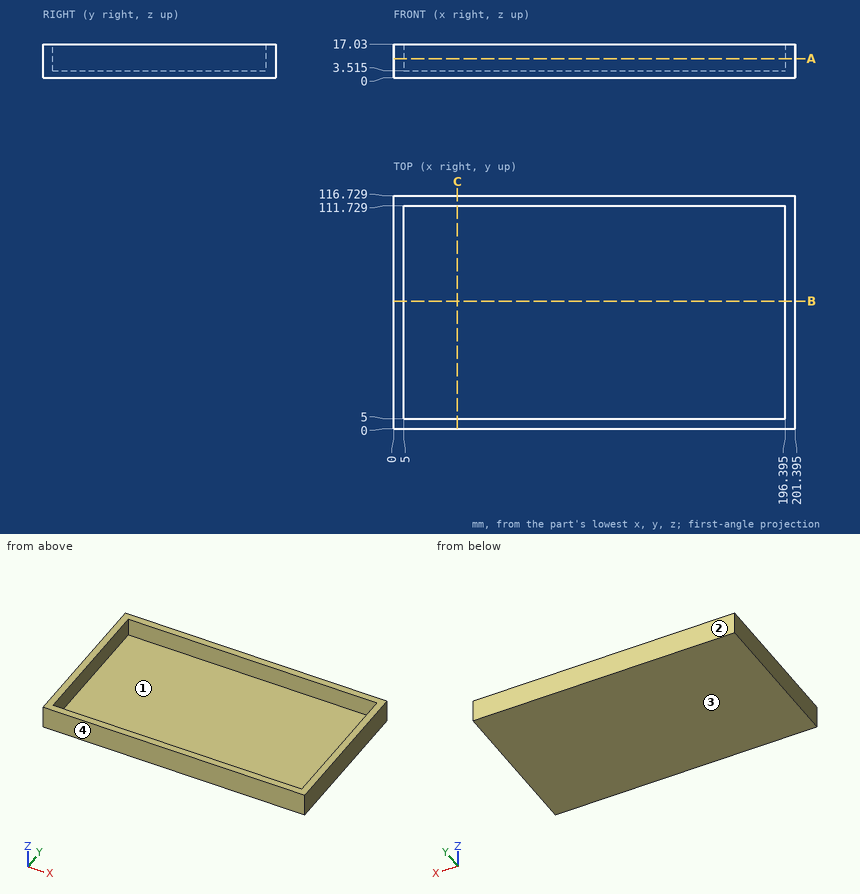
Check sheet for the drawn part. Datum: minimum x, y, z corner. Units: mm. Give positions to 0.01 mm unless a question says otherwise; leave off trailing zeros. Loops run counter-clockwise (first coordinate to the right, second up) from the corner with the lowest first, then second, coordinate; pieces in that order, holes last. Notation, with made-up numbers: M -16,50.25 L -2,50.25 A20 ccw -2,59.25 Z; hole C 40.25,33.5 d8. An arc over 180 degrees is marked long. Return JSON: item names as keys, results as strings.
1) Material ranges on L1, parallel to Y at x = 171, z = 12.25; L2, parallel to X at y = 99, z = 16.25 (3 decimals); L3, parallel to Z at x = 111, y = 43.5 (3 decimals), recorded low to high. Write a range as [from, to].
Findings:
{"L1": "y = [0, 5], [111.73, 116.73]", "L2": "x = [0, 5], [196.395, 201.395]", "L3": "z = [0, 3.515]"}
2) Section check B-B, the plane y = 64. Enter the section's corners in (x, z) (3 decimals).
Findings:
{"outline": "M 0,0 L 201.395,0 L 201.395,17.03 L 196.395,17.03 L 196.395,3.515 L 5,3.515 L 5,17.03 L 0,17.03 Z"}
3) Section check C-C, the plane x = 32. Enter the section's corners in (y, z) (3 decimals), and give its area (3 significant figures).
Findings:
{"outline": "M 0,0 L 116.729,0 L 116.729,17.03 L 111.729,17.03 L 111.729,3.515 L 5,3.515 L 5,17.03 L 0,17.03 Z", "area": "545 mm2"}
4) Gauge pin test, flat end, axial feed: P1, Ø1.5, axis at x = 167.5, y = 104.5, coming from the -Z side. Record the tip position at first contact, or that the pin passes through.
Findings:
{"P1": "stops at z = 0"}
5) Mould release check, pull along Y, two halves, no side actions. Record for the marked faces 1, 2, 3 and 4: released by +Y, released by -Y, zero draft, split by the parting line, or undercut.
Findings:
{"face 1": "undercut", "face 2": "released by +Y", "face 3": "zero draft", "face 4": "released by -Y"}
6) Section check A-A, the plane z = 9.75. Enter the section's corners in (x, y) (3 decimals), and give its area (3 significant figures).
Findings:
{"outline": "M 0,0 L 201.395,0 L 201.395,116.729 L 0,116.729 Z; hole M 5,5 L 196.395,5 L 196.395,111.729 L 5,111.729 Z", "area": "3,080 mm2"}
